The listing builds one solid part. Answer for the finished solid, in the listing's coordinates (mm). Coordinates: 2 decimals unless noted, no trailing zeros. Order: outer loops, then holes, each group sorted by start corner. A loop starts at its lowest first (then second) coordinate and runs counter-clockwise, first axis right, second up. Notation, with made-up numbers: (28, 16.5) -> (66, 16.5) arc R24 ccw to (66, 31.5) -> close; hole circle Ø5 at (-23.75, -9). An arc over 180 degrees is marked (long way). Answer in a Markdown table with one row per item.
```python
from build123d import *

# Parameters (mm, degrees)
TORUS_R           = 1
TORUS001_R        = 1
CYLINDER001_R     = 10.4
CYLINDER001_DEPTH = 130
CYLINDER_R        = 12.5
CYLINDER_DEPTH    = 130


with BuildPart() as torus:
    # Torus → Torus (revolve)
    with BuildSketch(Plane(origin=(0, 0, 55), x_dir=(1, 0, 0), z_dir=(0, -1, 0))):
        with Locations((13, 0)):
            Circle(TORUS_R)
    revolve(axis=Axis((0, 0, 55), (0, 0, 1)))


with BuildPart() as torus001:
    # Torus001 → Torus001 (revolve)
    with BuildSketch(Plane(origin=(0, 0, 50), x_dir=(1, 0, 0), z_dir=(0, -1, 0))):
        with Locations((13, 0)):
            Circle(TORUS001_R)
    revolve(axis=Axis((0, 0, 50), (0, 0, 1)))


with BuildPart() as cylinder001:
    # Cylinder001 → Cylinder001 (new body)
    with BuildSketch(Plane.XY):
        Circle(CYLINDER001_R)
    extrude(amount=CYLINDER001_DEPTH)


with BuildPart() as cut002:
    # Cylinder → Cylinder (new body)
    with BuildSketch(Plane.XY):
        Circle(CYLINDER_R)
    extrude(amount=CYLINDER_DEPTH)

    # Cut: cut Cylinder001
    add(cylinder001.part, mode=Mode.SUBTRACT)

    # Cut001: cut Torus001
    add(torus001.part, mode=Mode.SUBTRACT)

    # Cut002: cut Torus
    add(torus.part, mode=Mode.SUBTRACT)


solid = cut002.part
```
(1) A cutting plane is placed at A-A, the plane x = 0. Determine the outline of the cut face in (y, z).
Check values:
| item | result |
|---|---|
| outline | (-12.5, 0) -> (-10.4, 0) -> (-10.4, 130) -> (-12.5, 130) -> (-12.5, 55.87) arc R1 cw to (-12.5, 54.13) -> (-12.5, 50.87) arc R1 cw to (-12.5, 49.13) -> close; (10.4, 0) -> (12.5, 0) -> (12.5, 49.13) arc R1 cw to (12.5, 50.87) -> (12.5, 54.13) arc R1 cw to (12.5, 55.87) -> (12.5, 130) -> (10.4, 130) -> close |
(2) A cutting plane is placed at C-C, the plane z = 65. Determine the outline of the cut face in (x, y), then the cut area to 3 significant figures.
Check values:
| item | result |
|---|---|
| outline | circle Ø25 at (0, 0); hole circle Ø20.8 at (0, 0) |
| area | 151 mm² |
(3) Flat-ended cylindrical pins translate along their axes: pin 1 (4 mm diameter, centred on x = -10, z = 77.5, fed in from +Y); pin 2 (12 mm diameter, centred on x = -1.5, y = 1.5, fed in from -Z); pin 3 (1 mm diameter, centred on y = 2, z = 44, fed in from +X); pin 4 (1 mm diameter, centred on x = 7, z = 99, fed in from +Y). Find the tip coordinate at first contact, or state that the pin passes through.
Check values:
| item | result |
|---|---|
| pin 1 | y = 9.6 |
| pin 2 | through |
| pin 3 | x = 12.41 |
| pin 4 | y = 10.68 |
(4) For a pull along Y with two mould halves and no side action, classify faces 1 (the cylindrical face through (-1.35, 10.31, 64.09)), 2 (the flat face through (-2.8, 10.2, 0)), 3 (the cylindrical face through (11.923, 3.755, 52.477)) as released by +Y, released by -Y, zero draft, split by the parting line, or undercut.
Check values:
| item | result |
|---|---|
| face 1 | undercut |
| face 2 | zero draft |
| face 3 | split by the parting line |
(5) Find the intervals of material crossed by line 1 along Y through (x, z) = (0, 64); line 2 along Z through (x, y) = (5.75, -11); line 3 along Y through (x, z) = (8.5, 56.5), in increasing order. Write a range as from..to.
Check values:
| item | result |
|---|---|
| line 1 | -12.5..-10.4, 10.4..12.5 |
| line 2 | 0..49.19, 50.81..54.19, 55.81..130 |
| line 3 | -9.17..-5.99, 5.99..9.17 |
